from build123d import *

# Parameters (mm, degrees)
FILETE3_R     = 4
CHANFRO7_SIZE = 2.7


with BuildPart() as part:
    # Esboço1 → Revolução1 (revolve)
    with BuildSketch(Plane.XY, mode=Mode.PRIVATE) as revolu_o1_sk:
        Polygon((0, 3.3), (0, 4), (4, 4.3), (10, 4.3), (17.4, 6.4), (58.4, 6.4), (58.4, 5), (63.4, 5), (63.4, 6.4), (68, 6.4), (68, 3.3), align=None)
    revolve(revolu_o1_sk.sketch.rotate(Axis((0, 0, 0), (1, 0, 0)), 90), axis=Axis((0, 0, 0), (1, 0, 0)))

    # Filete3
    # the kernel refuses this fillet: 4 mm, written as the material it takes off along each edge
    with BuildSketch(Plane(origin=(0, 0, 0), x_dir=(0, 0, 1), z_dir=(0, 1, 0))) as filete3_piece_1:
        with BuildLine():
            CenterArc((0.176138028, 2.498296696), FILETE3_R, 321.349060222, 34.361786449)
            Line((4.164935268, 2.199136903), (4.244711213, 2.193153707))
            Line((4.244711213, 2.193153707), (4.079775945, -0.005983196))
            Line((4.079775945, -0.005983196), (4, -0.08))
            ThreePointArc((4, -0.08), (3.65, -0.08), (3.362477239, -0.049965934))
            Line((3.362477239, -0.049965934), (3.3, 0))
        make_face()
    revolve(axis=Axis((0, 0, 0), (1, 0, 0)), mode=Mode.SUBTRACT)

    # Chanfro7
    chanfro7_edges = [part.edges().sort_by_distance(p)[0] for p in [
        (68, 0, -3.3),
    ]]
    chamfer(chanfro7_edges, length=CHANFRO7_SIZE)


solid = part.part
Model file for the job. Use its own axes, mm. A direction names the side the tool comes from. Round coordinates to 2 decimals unless told otherwise and drop trailing zeros. Loops run counter-clockwise (first coordinate to the right, second up) from the corner with the lowest first, then second, coordinate; pieces in that order, holes last. Notation, with made-up numbers: (0, 53.5) -> (25, 53.5) arc R31 cw to (25, 87.5) -> close; hole circle Ø11 at (32.25, 38). An arc over 180 degrees is marked (long way). Answer as CSV lines item,"result". Start each with the question number.
1) Slice it at A-A (x = 62). List the corners of the cut face in (y, z), plus the area to 3 significant figures.
2) Tool access for faces 1 (the face through (65.732, -1.922, 6.104)), 2 (the face through (7.042, -0.189, -4.296)), 3 (the face through (61, 0, -5)): list every direction of +Z, -Z, +X, -X, +Y, -Y with a clear straight run to the whole face (end or side of a thin tool).
3) Mould opens along Z. For faces 4 (the face through (2.71, 3.73, 1.94)), 5 (the face through (32.19, -2.23, -2.43)), 6 (the face through (63.4, 2, 5)) say: +Z half, -Z half, draft (parallel to the pull), parting line (faces both ways), or undercut.
4) Slice it at B-B (x = 19.5). List the corners of the cut face in (y, z).
5) Pin check, flat tips, straight feed: P1, Ø6, axis at y = 0, z = 0, coming from the +X side; P2, Ø2, axis at y = -1, z = 4, coming from the -X side; P3, Ø4, axis at x = 55.5, z = -4.5, coming from the -Y side; P4, Ø1, axis at x = 20.5, z = 3, coming from the +Y side. Stop position of each tip, or through.
6) Probe line 1 along Y through (x, z) = (22, 0); line 2 along Z through (x, y) = (34, 1); line 3 along Y through (x, z) = (55.5, 0.75). List the from-to ranges inside material, lowest first.
Filled in:
1,outline,"circle Ø10 at (0, 0); hole circle Ø6.6 at (0, 0)"
1,area,"44.3 mm2"
2,face 1,"+X, -X"
2,face 2,"-X"
2,face 3,"none"
3,face 4,"parting line"
3,face 5,"undercut"
3,face 6,"draft"
4,outline,"circle Ø12.8 at (0, 0); hole circle Ø6.6 at (0, 0)"
5,P1,"passes through"
5,P2,"stops at x = 0"
5,P3,"stops at y = -5.89"
5,P4,"stops at y = 5.89"
6,line 1,"y = -6.4 to -3.3, 3.3 to 6.4"
6,line 2,"z = -6.32 to -3.14, 3.14 to 6.32"
6,line 3,"y = -6.36 to -3.21, 3.21 to 6.36"
